Input: part model. Units: mm. Frame: model coordinates. Give positions to 0.01 mm unless a question says otherwise; leave off trailing zeros. Loops run counter-clockwise (first coordinate to the right, second up) from the corner with the lowest first, then second, coordinate; pieces in that order, holes last. Notation, with made-up numbers: (83, 49) - (134, 49) arc R8 cw to (134, 60) - close; hole circle Ø11 at (-19.5, -24). An arc over 180 degrees is marked (long way). Answer as a JSON object with one key per item and string values. Group by question number.
(1) Mould query, pull axis Y, two halves, no side actions, for faces 1 (the flat face through (-1, 1, 0)), 2 (the flat face through (-40.34, 59.74, 0.79)), 3 (the cylindrical face through (-44.708, 18.643, 0.789)), 4 (the flat face through (40.34, -59.74, 0.79)). Classes: +Y half, -Y half, draft (parallel to the pull), parting line (faces both ways), or undercut.
(2) Section query A-A (z = 0.95). Count the separate pieces of the cut face and the enclosed holes in it, plus the area to 3 significant figures.
(3) Section query B-B (x = -44.5). Return loops of the section in (y, z), plus the area to 3 significant figures.
(4) Material intervals for L1, parallel to X at y = 38, z = 1; L2, parallel to Y at x = 44.5, z = 0.6; L3, parallel to X at y = 52, z = 1.55, sorted ascending.
```python
from build123d import *

# Parameters (mm, degrees)
SKETCH_1_R      = 1.6
EXTRUDE_1_DEPTH = 1.6


with BuildPart() as part:
    # Эскиз1 → Бобышка-Вытянуть1 (new body)
    with BuildSketch(Plane.XY):
        with BuildLine():
            Line((33.914602025, -64.162611141), (46.943320266, -55.194045236))
            ThreePointArc((46.943320266, -55.194045236), (48.454507775, -53.491550465), (49, -51.281434095))
            Line((49, -51.281434095), (49, 51.281434095))
            ThreePointArc((49, 51.281434095), (48.454507775, 53.491550465), (46.943320266, 55.194045236))
            Line((46.943320266, 55.194045236), (33.914602025, 64.162611141))
            ThreePointArc((33.914602025, 64.162611141), (32.631529446, 64.785824232), (31.221281759, 65))
            Line((31.221281759, 65), (-31.221281759, 65))
            ThreePointArc((-31.221281759, 65), (-32.631529446, 64.785824232), (-33.914602025, 64.162611141))
            Line((-33.914602025, 64.162611141), (-46.943320266, 55.194045236))
            ThreePointArc((-46.943320266, 55.194045236), (-48.454507775, 53.491550465), (-49, 51.281434095))
            Line((-49, 51.281434095), (-49, -51.281434095))
            ThreePointArc((-49, -51.281434095), (-48.454507775, -53.491550465), (-46.943320266, -55.194045236))
            Line((-46.943320266, -55.194045236), (-33.914602025, -64.162611141))
            ThreePointArc((-33.914602025, -64.162611141), (-32.631529446, -64.785824232), (-31.221281759, -65))
            Line((-31.221281759, -65), (31.221281759, -65))
            ThreePointArc((31.221281759, -65), (32.631529446, -64.785824232), (33.914602025, -64.162611141))
        make_face()
        with Locations((44.5, 17.056509603)):
            Circle(SKETCH_1_R, mode=Mode.SUBTRACT)
        with Locations((-44.5, -17.056509603)):
            Circle(SKETCH_1_R, mode=Mode.SUBTRACT)
        with Locations((-44.5, 17.056509603)):
            Circle(SKETCH_1_R, mode=Mode.SUBTRACT)
        with Locations((-44.5, 38.056509603)):
            Circle(SKETCH_1_R, mode=Mode.SUBTRACT)
        with Locations((-44.5, -38.056509603)):
            Circle(SKETCH_1_R, mode=Mode.SUBTRACT)
        with Locations((44.5, -17.056509603)):
            Circle(SKETCH_1_R, mode=Mode.SUBTRACT)
        with Locations((44.5, -38.056509603)):
            Circle(SKETCH_1_R, mode=Mode.SUBTRACT)
        with Locations((44.5, 38.056509603)):
            Circle(SKETCH_1_R, mode=Mode.SUBTRACT)
    extrude(amount=EXTRUDE_1_DEPTH)


solid = part.part
```
Recorded:
{
 "1": {"face 1": "draft", "face 2": "+Y half", "face 3": "undercut", "face 4": "-Y half"},
 "2": {"separate pieces": "1", "enclosed holes": "8", "area": "12,300 mm^2"},
 "3": {"outline": "(-56.88, 0) - (-39.66, 0) - (-39.66, 1.6) - (-56.88, 1.6) - close; (-36.46, 0) - (-18.66, 0) - (-18.66, 1.6) - (-36.46, 1.6) - close; (-15.46, 0) - (15.46, 0) - (15.46, 1.6) - (-15.46, 1.6) - close; (18.66, 0) - (36.46, 0) - (36.46, 1.6) - (18.66, 1.6) - close; (39.66, 0) - (56.88, 0) - (56.88, 1.6) - (39.66, 1.6) - close", "area": "162 mm^2"},
 "4": {"L1": "x = -49 to -46.1, -42.9 to 42.9, 46.1 to 49", "L2": "y = -56.88 to -39.66, -36.46 to -18.66, -15.46 to 15.46, 18.66 to 36.46, 39.66 to 56.88", "L3": "x = -48.95 to 48.95"}
}
